For this review, take the finished solid that the model builds, in its own axes (mm). A direction names the side the tool comes from. Coordinates: 2 decimals unless noted, no trailing zeros. Order: outer loops, then holes, each group sorted by start corner. A loop starts at its lowest first (then second) coordinate and runs counter-clockwise, first axis right, second up.
from build123d import *

# Parameters (mm, degrees)
SM_START                         = -1
SM_BASE_FLANGE_1_DEPTH           = 1
SM_EDGE_FLANGE_1_STRIP_W         = 5.4732
SM_EDGE_FLANGE_1_STRIP_H         = 1
SM_EDGE_FLANGE_1_STRIP_CUT_DEPTH = 243.159735698
SM_EDGE_FLANGE_1_DEPTH           = 243.159735698
SM_EDGE_FLANGE_2_STRIP_W         = 5.4732
SM_EDGE_FLANGE_2_STRIP_H         = 1
SM_EDGE_FLANGE_2_STRIP_CUT_DEPTH = 99.02081528
SM_EDGE_FLANGE_2_DEPTH           = 99.02081528
SM_EDGE_FLANGE_3_STRIP_W         = 5.4732
SM_EDGE_FLANGE_3_STRIP_H         = 1
SM_EDGE_FLANGE_3_STRIP_CUT_DEPTH = 99.02081528
SM_EDGE_FLANGE_3_DEPTH           = 99.02081528
SM_EDGE_FLANGE_4_STRIP_W         = 5.4732
SM_EDGE_FLANGE_4_STRIP_H         = 1
SM_EDGE_FLANGE_4_STRIP_CUT_DEPTH = 243.159735698
SM_EDGE_FLANGE_4_DEPTH           = 243.159735698
CUT_EXTRUDE_1_REACH              = 277.58
SKETCH_18_R                      = 16.639768722


# Read off the part's stored shape, not the designer's step: Базовая кромка1
# Sheet-metal steps are written as plain solids
with BuildPart() as part:
    # Базовая кромка1 outline → Базовая кромка1 (new body)
    with BuildSketch(Plane.XY.offset(SM_START)):
        Polygon((-121.579867849, 49.51040764), (-125.579867849, 49.51040764), (-125.579867849, -49.51040764), (-121.579867849, -49.51040764), (-121.579867849, -53.51040764), (121.579867849, -53.51040764), (121.579867849, -49.51040764), (125.579867849, -49.51040764), (125.579867849, 49.51040764), (121.579867849, 49.51040764), (121.579867849, 53.51040764), (-121.579867849, 53.51040764), align=None)
    extrude(amount=SM_BASE_FLANGE_1_DEPTH)

    # Ребро-кромка1 strip (across the edge) → Ребро-кромка1 strip cut (cut)
    with BuildSketch(Plane(origin=(-121.579867849, 53.51040764, -1), x_dir=(0, -1, 0), z_dir=(1, 0, 0))):
        with Locations((-1, -0.5)):
            Rectangle(SM_EDGE_FLANGE_1_STRIP_W, SM_EDGE_FLANGE_1_STRIP_H)
    extrude(amount=SM_EDGE_FLANGE_1_STRIP_CUT_DEPTH, mode=Mode.SUBTRACT)

    # Ребро-кромка1 section (across the edge) → Ребро-кромка1 (add)
    with BuildSketch(Plane(origin=(-121.579867849, 53.51040764, -1), x_dir=(0, -1, 0), z_dir=(1, 0, 0))):
        with BuildLine():
            Line((0, 0.7366), (0, 99))
            Line((0, 99), (1, 99))
            Line((1, 99), (1, 0.7366))
            ThreePointArc((1, 0.7366), (1.215745145, 0.215745145), (1.7366, 0))
            Line((1.7366, 0), (1.7366, -1))
            ThreePointArc((1.7366, -1), (0.508638364, -0.491361636), (0, 0.7366))
        make_face()
    extrude(amount=SM_EDGE_FLANGE_1_DEPTH)

    # Ребро-кромка2 strip (across the edge) → Ребро-кромка2 strip cut (cut)
    with BuildSketch(Plane(origin=(-125.579867849, -49.51040764, -1), x_dir=(1, 0, 0), z_dir=(0, 1, 0))):
        with Locations((-1, -0.5)):
            Rectangle(SM_EDGE_FLANGE_2_STRIP_W, SM_EDGE_FLANGE_2_STRIP_H)
    extrude(amount=SM_EDGE_FLANGE_2_STRIP_CUT_DEPTH, mode=Mode.SUBTRACT)

    # Ребро-кромка2 section (across the edge) → Ребро-кромка2 (add)
    with BuildSketch(Plane(origin=(-125.579867849, -49.51040764, -1), x_dir=(1, 0, 0), z_dir=(0, 1, 0))):
        with BuildLine():
            Line((0, 0.7366), (0, 99))
            Line((0, 99), (1, 99))
            Line((1, 99), (1, 0.7366))
            ThreePointArc((1, 0.7366), (1.215745145, 0.215745145), (1.7366, 0))
            Line((1.7366, 0), (1.7366, -1))
            ThreePointArc((1.7366, -1), (0.508638364, -0.491361636), (0, 0.7366))
        make_face()
    extrude(amount=SM_EDGE_FLANGE_2_DEPTH)

    # Ребро-кромка3 strip (across the edge) → Ребро-кромка3 strip cut (cut)
    with BuildSketch(Plane(origin=(125.579867849, 49.51040764, -1), x_dir=(-1, 0, 0), z_dir=(0, -1, 0))):
        with Locations((-1, -0.5)):
            Rectangle(SM_EDGE_FLANGE_3_STRIP_W, SM_EDGE_FLANGE_3_STRIP_H)
    extrude(amount=SM_EDGE_FLANGE_3_STRIP_CUT_DEPTH, mode=Mode.SUBTRACT)

    # Ребро-кромка3 section (across the edge) → Ребро-кромка3 (add)
    with BuildSketch(Plane(origin=(125.579867849, 49.51040764, -1), x_dir=(-1, 0, 0), z_dir=(0, -1, 0))):
        with BuildLine():
            Line((0, 0.7366), (0, 99))
            Line((0, 99), (1, 99))
            Line((1, 99), (1, 0.7366))
            ThreePointArc((1, 0.7366), (1.215745145, 0.215745145), (1.7366, 0))
            Line((1.7366, 0), (1.7366, -1))
            ThreePointArc((1.7366, -1), (0.508638364, -0.491361636), (0, 0.7366))
        make_face()
    extrude(amount=SM_EDGE_FLANGE_3_DEPTH)

    # Ребро-кромка4 strip (across the edge) → Ребро-кромка4 strip cut (cut)
    with BuildSketch(Plane(origin=(121.579867849, -53.51040764, -1), x_dir=(0, 1, 0), z_dir=(-1, 0, 0))):
        with Locations((-1, -0.5)):
            Rectangle(SM_EDGE_FLANGE_4_STRIP_W, SM_EDGE_FLANGE_4_STRIP_H)
    extrude(amount=SM_EDGE_FLANGE_4_STRIP_CUT_DEPTH, mode=Mode.SUBTRACT)

    # Ребро-кромка4 section (across the edge) → Ребро-кромка4 (add)
    with BuildSketch(Plane(origin=(121.579867849, -53.51040764, -1), x_dir=(0, 1, 0), z_dir=(-1, 0, 0))):
        with BuildLine():
            Line((0, 0.7366), (0, 99))
            Line((0, 99), (1, 99))
            Line((1, 99), (1, 0.7366))
            ThreePointArc((1, 0.7366), (1.215745145, 0.215745145), (1.7366, 0))
            Line((1.7366, 0), (1.7366, -1))
            ThreePointArc((1.7366, -1), (0.508638364, -0.491361636), (0, 0.7366))
        make_face()
    extrude(amount=SM_EDGE_FLANGE_4_DEPTH)

    # Эскиз18 → Вырез-Вытянуть1 (cut, up to next)
    with BuildSketch(Plane.ZY.offset(125.579867849), mode=Mode.PRIVATE) as cut_extrude_1_sk1:
        with Locations((-67.065719066, -8.85501242)):
            Circle(SKETCH_18_R)
    cut_extrude_1_tool1 = extrude(cut_extrude_1_sk1.sketch, amount=-CUT_EXTRUDE_1_REACH, mode=Mode.PRIVATE) & part.part
    add(cut_extrude_1_tool1.solids().sort_by_distance((-125.579868, -8.855012, -67.065719))[0], mode=Mode.SUBTRACT)


solid = part.part
1. The part is to be moulded in two halves that separate along X. For faces 4 (the face through (-125.58, -1, -50)), 5 (the face through (125.58, 1, -50)), 6 (the face through (-2, 1, -1)), 7 (the face through (-125.09, -8.12, -83.69)), say which applies: +X half, -X half, draft (parallel to the pull), parting line (faces both ways), or undercut.
Answer below:
face 4: -X half
face 5: +X half
face 6: undercut
face 7: draft
2. Take a section at D-D, the plane x = -102. Give the boundary of the cut face in (y, z).
Answer below:
outline: (-53.51, -100) - (-52.51, -100) - (-52.51, -1.74) arc R0.74 cw to (-51.77, -1) - (51.77, -1) arc R0.74 cw to (52.51, -1.74) - (52.51, -100) - (53.51, -100) - (53.51, -1.74) arc R1.74 ccw to (51.77, 0) - (-51.77, 0) arc R1.74 ccw to (-53.51, -1.74) - close
3. Take a section at A-A, the plane z = -41. Give the boundary of the cut face in (x, y).
Answer below:
outline: (-125.58, -49.51) - (-124.58, -49.51) - (-124.58, 49.51) - (-125.58, 49.51) - close; (-121.58, -53.51) - (121.58, -53.51) - (121.58, -52.51) - (-121.58, -52.51) - close; (-121.58, 52.51) - (121.58, 52.51) - (121.58, 53.51) - (-121.58, 53.51) - close; (124.58, -49.51) - (125.58, -49.51) - (125.58, 49.51) - (124.58, 49.51) - close
4. Take a section at B-B, the plane y = -44. Give the boundary of the cut face in (x, z), plus the area to 3 significant figures.
Answer below:
outline: (-125.58, -100) - (-124.58, -100) - (-124.58, -1.74) arc R0.74 cw to (-123.84, -1) - (123.84, -1) arc R0.74 cw to (124.58, -1.74) - (124.58, -100) - (125.58, -100) - (125.58, -1.74) arc R1.74 ccw to (123.84, 0) - (-123.84, 0) arc R1.74 ccw to (-125.58, -1.74) - close
area: 448 mm2
5. Machinability: for faces 1 (the face through (2, -52.51, -52)), 2 (the face through (-124.58, -1, -52)), 3 (the face through (2, -53.51, -50)), which of the approach directions +Z, -Z, +X, -X, +Y, -Y give a long, thin tool a straight path to every point of the face, cutting with its end or side? Answer none if there is none.
Answer below:
face 1: -Z, +X, -X
face 2: -Z, +Y, -Y
face 3: +Z, -Z, +X, -X, -Y
6. Clearance check with flat-ended pins moving along their axes: pin 1 Ø3 at (y, z) = (52, -26.5) entering from -X; pin 2 Ø1.5 at (x, y) = (93.5, 3) entering from -Z; pin 3 Ø1.2 at (y, z) = (-52.5, -60) entering from +X. State where each tip first meets the part, or that it passes through.
Answer below:
pin 1: stops at x = -121.58
pin 2: stops at z = -1
pin 3: stops at x = 121.58
7. To check wall thickness, follow L1, parallel to Y at x = -31, z = -79; L2, parallel to X at y = 39, z = -69; L3, parallel to Z at x = 108.5, y = -15.5. State the ranges of each line that lie inside material, in increasing order.
Answer below:
L1: y = -53.51 to -52.51, 52.51 to 53.51
L2: x = -125.58 to -124.58, 124.58 to 125.58
L3: z = -1 to 0
8. Take a section at C-C, the plane y = -1. Give the boundary of the cut face in (x, z).
Answer below:
outline: (-125.58, -100) - (-124.58, -100) - (-124.58, -81.73) - (-125.58, -81.73) - close; (-125.58, -52.4) - (-124.58, -52.4) - (-124.58, -1.74) arc R0.74 cw to (-123.84, -1) - (123.84, -1) arc R0.74 cw to (124.58, -1.74) - (124.58, -100) - (125.58, -100) - (125.58, -1.74) arc R1.74 ccw to (123.84, 0) - (-123.84, 0) arc R1.74 ccw to (-125.58, -1.74) - close
